from build123d import *

# Parameters (mm, degrees)
F0_W          = 206
F0_H          = 56
F1_DEPTH      = 13
F2_T          = -3
F4_DEPTH      = 10
F5_W          = 8
F5_H          = 13
F6_DEPTH      = 6
F7_W          = 8
F7_H          = 6
F8_DEPTH      = 3
F9_R          = 2.99999
F11_D         = 3
F12_W         = 5.25
F12_H         = 1
F13_DEPTH     = 3
F14_T1_DEPTH  = 5.5
F14_T3_DEPTH  = 4.1572120132
F14_T5_DEPTH  = 3.75
F14_T7_DEPTH  = 6
F14_T9_DEPTH  = 3.25
F14_T11_DEPTH = 2.5
F14_T13_DEPTH = 1
F14_S17_W     = 0.5
F14_S17_H     = 0.5
F14_T18_DEPTH = 0.5
F14_S23_W     = 0.5
F14_S23_H     = 0.5
F14_T24_DEPTH = 0.5
F14_S29_W     = 0.5
F14_S29_H     = 0.5
F14_T30_DEPTH = 0.5
F14_T36_DEPTH = 1.6727936268


# Not quite as in the source:
# - a fillet or chamfer that OpenCascade refuses, or shapes differently, is made with other operations: its cross-section is extruded or revolved along the edge and cut away or added
# - a fillet or chamfer is up to 0.001 mm smaller than in the source, because OpenCascade refuses the exact size


with BuildPart() as f1:
    # F0 (on Top) → F1 (new body)
    with BuildSketch(Plane.XY):
        Rectangle(F0_W, F0_H)
    extrude(amount=F1_DEPTH)

    # F2
    f2_openings = [f1.faces().sort_by_distance(p)[0] for p in [
        (0, 0, 13),
    ]]
    offset(amount=F2_T, openings=f2_openings)

    # F3 (on face) → F4 (join)
    with BuildSketch(Plane.XY.offset(3)):
        Polygon((100, 11.5), (-100, -8.5), (-100, -11.5), (100, 8.5), align=None)
    extrude(amount=F4_DEPTH)

    # F5 (on face) → F6 (join)
    with BuildSketch(Plane(origin=(0, 28, 0), x_dir=(-1, 0, 0), z_dir=(0, 1, 0))):
        with Locations((-74, 6.5)):
            Rectangle(F5_W, F5_H)
        with Locations((74, 6.5)):
            Rectangle(F5_W, F5_H)
    extrude(amount=F6_DEPTH)

    # F7 (on face) → F8 (join)
    with BuildSketch(Plane.XY.offset(13)):
        with Locations((-74, 31)):
            Rectangle(F7_W, F7_H)
        with Locations((74, 31)):
            Rectangle(F7_W, F7_H)
    extrude(amount=F8_DEPTH)

    # F9 (radius 3 in the source; OpenCascade refuses exactly that, so slightly less here)
    f9_edges = [f1.edges().sort_by_distance(p)[0] for p in [
        (-74, 28, 16),
        (-74, 34, 16),
        (74, 34, 16),
        (74, 28, 16),
    ]]
    fillet(f9_edges, radius=F9_R)

    # F11 (through all)
    with Locations(Plane.YZ.offset(78)):
        with Locations((31, 13)):
            Hole(F11_D / 2)

    # F12 (on face) → F13 (join)
    with BuildSketch(Plane.XZ.offset(28)):
        Polygon((-0.75, 12.9227936268), (0.25, 13), (-5, 13), (-5, 12), (-0.75, 12), align=None)
        with Locations((-2.375, 13.5)):
            Rectangle(F12_W, F12_H)
    extrude(amount=F13_DEPTH)

    # F14: fillet of radius 0.5 on 9 edges, made by hand

    # F14_s2 → F14_t1 (cut)
    with BuildSketch(Plane.XZ.offset(26.75)):
        with BuildLine():
            ThreePointArc((0.25, 13.5), (0.1035533906, 13.8535533906), (-0.25, 14))
            Line((-0.25, 14), (0.25, 14))
            Line((0.25, 14), (0.25, 13.5))
        make_face()
    extrude(amount=F14_T1_DEPTH, mode=Mode.SUBTRACT)

    # F14_s4 → F14_t3 (cut)
    with BuildSketch(Plane.XZ.offset(28)):
        with BuildLine():
            ThreePointArc((-0.211511355, 12.9643683821), (0.1169089277, 13.1232116701), (0.25, 13.4628848053))
            Line((0.25, 13.4628848053), (0.25, 13))
            Line((0.25, 13), (-0.211511355, 12.9643683821))
        make_face()
    extrude(amount=F14_T3_DEPTH, mode=Mode.SUBTRACT)

    # F14_s6 → F14_t5 (cut)
    with BuildSketch(Plane.XZ.offset(26.75)):
        with BuildLine():
            ThreePointArc((-5, 13.5), (-4.8535533906, 13.8535533906), (-4.5, 14))
            Line((-4.5, 14), (-5, 14))
            Line((-5, 14), (-5, 13.5))
        make_face()
    extrude(amount=F14_T5_DEPTH, mode=Mode.SUBTRACT)

    # F14_s8 → F14_t7 (cut)
    with BuildSketch(Plane.YZ.offset(-4.5)):
        with BuildLine():
            ThreePointArc((-31, 13.5), (-30.8535533906, 13.8535533906), (-30.5, 14))
            Line((-30.5, 14), (-31, 14))
            Line((-31, 14), (-31, 13.5))
        make_face()
    extrude(amount=F14_T7_DEPTH, mode=Mode.SUBTRACT)

    # F14_s10 → F14_t9 (cut)
    with BuildSketch(Plane.YZ.offset(-4.5)):
        with BuildLine():
            ThreePointArc((-30.5, 12), (-30.8535533906, 12.1464466094), (-31, 12.5))
            Line((-31, 12.5), (-31, 12))
            Line((-31, 12), (-30.5, 12))
        make_face()
    extrude(amount=F14_T9_DEPTH, mode=Mode.SUBTRACT)

    # F14_s12 → F14_t11 (cut)
    with BuildSketch(Plane.XZ.offset(28)):
        with BuildLine():
            ThreePointArc((-0.75, 12.5), (-0.8964466094, 12.1464466094), (-1.25, 12))
            Line((-1.25, 12), (-0.75, 12))
            Line((-0.75, 12), (-0.75, 12.5))
        make_face()
        with BuildLine():
            ThreePointArc((-4.5, 12), (-4.8535533906, 12.1464466094), (-5, 12.5))
            Line((-5, 12.5), (-5, 12))
            Line((-5, 12), (-4.5, 12))
        make_face()
    extrude(amount=F14_T11_DEPTH, mode=Mode.SUBTRACT)

    # F14_s14 → F14_t13 (cut)
    with BuildSketch(Plane.XY.offset(12.5)):
        with BuildLine():
            ThreePointArc((-5, -30.5), (-4.8535533906, -30.8535533906), (-4.5, -31))
            Line((-4.5, -31), (-5, -31))
            Line((-5, -31), (-5, -30.5))
        make_face()
    extrude(amount=F14_T13_DEPTH, mode=Mode.SUBTRACT)


with BuildPart() as f14_tool16:
    # F14_s17 → F14_t18 (new body)
    with BuildSketch(Plane.YZ.offset(-4.5)):
        with Locations((-30.75, 13.75)):
            Rectangle(F14_S17_W, F14_S17_H)
    extrude(amount=-F14_T18_DEPTH)

    # F14_s19 → F14_t20 (revolve, cut)
    with BuildSketch(Plane(origin=(-4.5, -30.5, 13.5), x_dir=(0, 0.7071067812, -0.7071067812), z_dir=(0, 0.7071067812, 0.7071067812))):
        with BuildLine():
            ThreePointArc((0, -0.5), (0.5, 0), (0, 0.5))
            Line((0, 0.5), (0, -0.5))
        make_face()
    revolve(axis=Axis((-4.5, -30.5, 13.5), (-1, 0, 0)), mode=Mode.SUBTRACT)


with BuildPart() as f1_1:
    add(f1.part)

    # F14_t15: cut F14_tool16
    add(f14_tool16.part, mode=Mode.SUBTRACT)


with BuildPart() as f14_tool22:
    # F14_s23 → F14_t24 (new body)
    with BuildSketch(Plane.XY.offset(12.5)):
        with Locations((-4.75, -30.75)):
            Rectangle(F14_S23_W, F14_S23_H)
    extrude(amount=-F14_T24_DEPTH)

    # F14_s25 → F14_t26 (revolve, cut)
    with BuildSketch(Plane(origin=(-4.5, -30.5, 12.5), x_dir=(0.7071067812, 0.7071067812, 0), z_dir=(-0.7071067812, 0.7071067812, 0))):
        with BuildLine():
            ThreePointArc((0, -0.5), (0.5, 0), (0, 0.5))
            Line((0, 0.5), (0, -0.5))
        make_face()
    revolve(axis=Axis((-4.5, -30.5, 12.5), (0, 0, -1)), mode=Mode.SUBTRACT)


with BuildPart() as f1_2:
    add(f1_1.part)

    # F14_t21: cut F14_tool22
    add(f14_tool22.part, mode=Mode.SUBTRACT)


with BuildPart() as f14_tool28:
    # F14_s29 → F14_t30 (new body)
    with BuildSketch(Plane.YZ.offset(-1.25)):
        with Locations((-30.75, 12.25)):
            Rectangle(F14_S29_W, F14_S29_H)
    extrude(amount=F14_T30_DEPTH)

    # F14_s31 → F14_t32 (revolve, cut)
    with BuildSketch(Plane(origin=(-1.25, -30.5, 12.5), x_dir=(0, 0.7071067812, 0.7071067812), z_dir=(0, 0.7071067812, -0.7071067812))):
        with BuildLine():
            ThreePointArc((0, -0.5), (0.5, 0), (0, 0.5))
            Line((0, 0.5), (0, -0.5))
        make_face()
    revolve(axis=Axis((-1.25, -30.5, 12.5), (1, 0, 0)), mode=Mode.SUBTRACT)


with BuildPart() as f1_3:
    add(f1_2.part)

    # F14_t27: cut F14_tool28
    add(f14_tool28.part, mode=Mode.SUBTRACT)


with BuildPart() as f14_tool34:
    # F14_s35 → F14_t36 (new body)
    with BuildSketch(Plane.XY.offset(12.5)):
        with BuildLine():
            ThreePointArc((-0.75, -30.5), (-0.8964466094, -30.8535533906), (-1.25, -31))
            Line((-1.25, -31), (-0.75, -31))
            Line((-0.75, -31), (-0.75, -30.5))
        make_face()
    extrude(amount=F14_T36_DEPTH)

    split(bisect_by=Plane(origin=(-0.9962541501, 0, 12.903781237), x_dir=(0, 1, 0), z_dir=(0.07697729, 0, -0.9970328464)), keep=Keep.TOP)


with BuildPart() as f1_4:
    add(f1_3.part)

    # F14_t33: cut F14_tool34
    add(f14_tool34.part, mode=Mode.SUBTRACT)


solid = f1_4.part
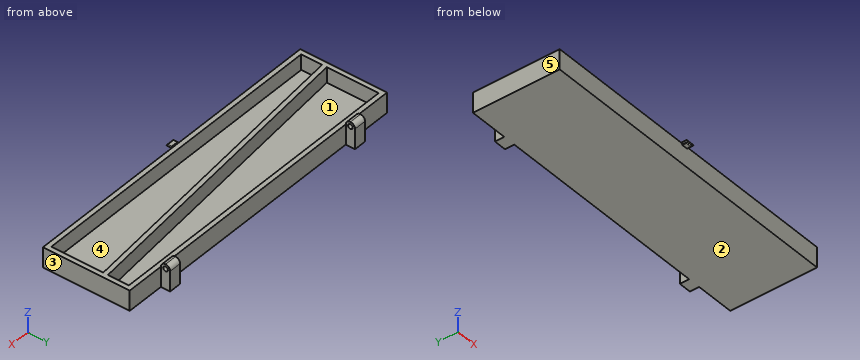
Check sheet for the modelled part. Datum: model origin and axes. Units: mm. Face numbers are marked on the shaded views. A direction names the side the tool comes from. Give positions to 0.01 mm unless a question says otherwise; leave off trailing zeros. Loops run counter-clockwise (first coordinate to the right, second up) from the corner with the lowest first, then second, coordinate; pieces in that order, holes last. Notation, with made-up numbers: M 4.5,-10 L 38.5,-10 A16 ccw 38.5,12 Z; hole C -29,45.25 d8. An arc over 180 degrees is marked long. Answer as a JSON object with one key per item and string values. Group by question number.
Q1. Cross-section at A-A on x = 84.5. Record the cut outline in (y, z).
Q2. Go/stop test with flat-tipped pins: P1, Ø6, axis at x = 62, z = 11, coming from the -Y side; P2, Ø4, axis at x = 89, z = 5.5, coming from the +Y side; P3, Ø0.8, axis at x = -3.5, y = -28.5, coming from the -Z side; P4, Ø2.5, axis at y = 31, z = 13, coming from the +X side. Record where each tip stops, or that it passes through.
Q3. Release check for a two-part mould opening along X. For the marked faces 1, 2 and 3 record: released by +X, released by -X, zero draft, split by the parting line, or undercut.
Q4. Cross-section at B-B on y = -2.5. Record the cut outline in (x, z).
Q5. Cross-section at C-C on y = -16.5. Record the cut outline in (x, z).
Q6. Material ranges on line 1 along X through (y, z) = (-18, 6); line 2 along Z through (x, y) = (76, 31); line 3 along Y through (x, z) = (73.5, 4), recorded low to high. Write a range as [from, to].
Q7. Access from +Z, -Z, +X, -X, +Y, -Y to the whole of each face (thin tool, end or side, straight path). Record for the marked faces 4 and 5.
Evaluation:
{
 "1": {"outline": "M -28,0 L 28,0 L 28,13 L 25,13 L 25,3 L 9.95,3 L 9.95,13 L 6.95,13 L 6.95,3 L -25,3 L -25,13 L -28,13 Z"},
 "2": {"P1": "stops at y = -28", "P2": "stops at y = 28", "P3": "stops at z = 12", "P4": "passes through"},
 "3": {"face 1": "undercut", "face 2": "zero draft", "face 3": "released by +X"},
 "4": {"outline": "M -103,0 L 103,0 L 103,13 L 100,13 L 100,3 L -10,3 L -10,13 L -40,13 L -40,3 L -100,3 L -100,13 L -103,13 Z"},
 "5": {"outline": "M -103,0 L 103,0 L 103,13 L 100,13 L 100,3 L -100,3 L -100,13 L -103,13 Z"},
 "6": {"line 1": "x = [-103, -100], [100, 103]", "line 2": "z = [0, 11.5], [14.5, 16]", "line 3": "y = [-28, -25], [5.85, 8.85], [25, 34]"},
 "7": {"face 4": "+Z", "face 5": "+Z, -Z, -X, +Y, -Y"}
}
